Autodesk Inventor part; units mm, degrees
ref_plane "Work Plane1" through (34.6079, -50.31, 0) normal (0, 0, 1) x (1, 0, 0)
ref_plane "YZ Plane" through (0, 0, 0) normal (1, 0, 0) x (0, 1, 0)
ref_plane "XZ Plane" through (0, 0, 0) normal (0, 1, 0) x (-1, 0, 0)
ref_plane "Work Plane1" through (34.6079, -50.31, 0) normal (0, 0, 1) x (1, 0, 0)
sketch "Sketch1" plane through (34.6079, -50.31, 0) normal (0, 0, 1) x (1, 0, 0)
  circle A0 centre (-188.0909, 15.5737) radius 4.445
  circle A1 centre (-194.7256, 7.071) radius 4.445
  circle A2 centre (-23.7989, 15.7765) radius 4.445
  circle A3 centre (-17.1643, 7.2737) radius 4.445
  line L0 (-188.0964, 20.0187) -> (-23.8044, 20.2215) construction
  line L1 (-48.7158, 54.9348) -> (8.8737, -18.8701)
  line L2 (-17.1592, 2.8288) -> (-194.7205, 2.626) construction
  line L3 (-163.0158, 54.9348) -> (-220.6053, -18.8701)
  line L4 (-174.2476, 54.9348) -> (-39.5273, 54.9348) construction
  line L5 (-163.0158, 54.9348) -> (-163.0158, 93.0348)
  line L6 (-163.0158, 93.0348) -> (-48.7158, 93.0348)
  line L7 (-48.7158, 93.0348) -> (-48.7158, 54.9348)
  line L8 (-286.9371, -18.8701) -> (2.6787, -18.8701)
  line L9 (-201.5553, 5.5438) -> (-201.5553, -18.8701)
  line L10 (-10.1763, 5.5438) -> (-10.1763, -18.8701)
  line L11 (-201.5553, -18.8701) -> (-201.5553, -25.2201)
  line L12 (-201.5553, -25.2201) -> (-10.1763, -25.2201)
  line L13 (-10.1763, -25.2201) -> (-10.1763, -18.8701)
  circle A4 centre (-194.7256, 7.071) radius 2.286
  circle A5 centre (-188.0909, 15.5737) radius 2.286
  circle A6 centre (-23.7989, 15.7765) radius 2.286
  circle A7 centre (-17.1643, 7.2737) radius 2.286
  circle A8 centre (-137.0599, 81.1641) radius 2.286
  circle A9 centre (-73.5599, 81.1641) radius 2.286
  point P0 (-34.6079, 50.31)
  point P1 (-20.2945, 18.5109)
  point P2 (-13.6599, 10.0082)
  point P3 (-191.5953, 18.3082)
  point P4 (-198.23, 9.8054)
  dimension "d0" = 8.89
  dimension "d1" = 8.89
  dimension "d2" = 8.89
  dimension "d3" = 8.89
  dimension "d6" = 114.3
  dimension "d7" = 38.1
  dimension "d10" = 19.05
  dimension "d11" = 19.05
  dimension "d12" = 6.35
extrude "Extrusion1" add sketch "Sketch1" along normal blind 3.175 contours A0 | A1 | A3 | A2 | L3 L5 L6 L7 L1 L10 L8 L9 | L8 L13 L12 L11
fillet "Fillet1" radius 3.175 4 edges at (-128.4079, 42.7248, 1.5875) (-14.1079, 42.7248, 1.5875) (-166.9474, -44.7663, 1.5875) (24.4315, -44.7663, 1.5875)
fillet "Fillet2" radius 6.35 2 edges at (-128.4079, 4.6248, 1.5875) (-14.1079, 4.6248, 1.5875)
fillet "Fillet3" radius 6.35 2 edges at (24.4315, -75.5302, 1.5875) (-166.9474, -75.5302, 1.5875)
properties part number "PolyRamp1" material "Polycarbonate, Smoke"
Geometry check sheet. Reference: the model listing, model coordinates, mm. Round coordinates to 2 decimals unless told otherwise and drop trailing zeros. Loops run counter-clockwise (first coordinate to the right, second up) from the corner with the lowest first, then second, coordinate; pieces in that order, holes last.
Item 1: Gauge pin test, flat ends, axial feed: pin 1 (6 mm diameter, centred on x = 10.81, y = -34.53, fed in from -Z); pin 2 (1.6 mm diameter, centred on y = 25, z = 1.5, fed in from +X); pin 3 (2.5 mm diameter, centred on x = 17.44, y = -43.04, fed in from +Z); pin 4 (1.6 mm diameter, centred on y = 17.5, z = 1, fed in from -X). Record the tip position at first contact, or that the pin passes through.
Item 2: Thickness scan on line 1 (Y direction, x = -17, z = 2.5); line 2 (X direction, y = 11, z = 0.3); line 3 (Y direction, x = 4, z = 2.4). Record the ranges inside material, lowest first.
Item 3: Cross-section at B-B on y = 16.5. Record the boundary of the cut face in (x, z) (3 decimals).
Item 4: Cross-section at A-A on z = 1.15. Count the separate pieces of the cut face and the enclosed holes in it, then the cut area to 3 significant figures.
Item 5: Cross-section at C-C on x = 3. Record the boundary of the cut face in (y, z) (3 decimals), then the cut area to 3 significant figures.
Item 6: Mould release check, pull along Y, two halves, no side actions. Record for faces 1 (the cylindrical face through (-160.415, -45.506, 1.565)), 2 (the cylindrical face through (-165.137, -73.621, 1.61)), 3 (the flat face through (-73, -29, 3.175)), 4 (the flat face through (5.24, -20.17, 1.57)): pulls with the +Y half, pulls with the -Y half, needs draft (parallel to the pull), parting line crosses it, or undercut.
Answer sheet:
1. pin 1: stops at z = 0
1. pin 2: stops at x = -14.11
1. pin 3: passes through
1. pin 4: stops at x = -128.41
2. line 1: y = -75.53 to 42.71
2. line 2: x = -128.41 to -14.11
2. line 3: y = -75.53 to -18.58
3. outline: (-128.408, 0) - (-14.108, 0) - (-14.108, 3.175) - (-128.408, 3.175) - close
4. separate pieces: 1
4. enclosed holes: 6
4. area: 17,700 mm2
5. outline: (-75.53, 0) - (-17.3, 0) - (-17.3, 3.175) - (-75.53, 3.175) - close
5. area: 185 mm2
6. face 1: undercut
6. face 2: pulls with the -Y half
6. face 3: needs draft
6. face 4: pulls with the +Y half
